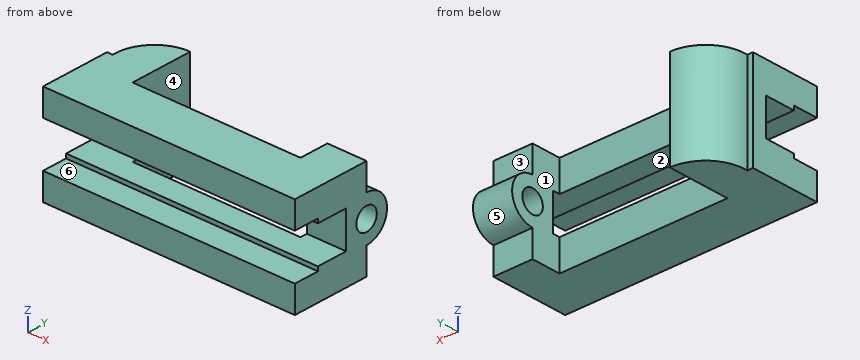
from build123d import *

# Parameters (mm, degrees)
BOSS_EXTRUDE1_DEPTH = 35
CUT_EXTRUDE1_DEPTH  = 201.062490237
SKETCH3_R           = 16
SKETCH3_R_2         = 8
BOSS_EXTRUDE2_DEPTH = 28
CUT_EXTRUDE2_REACH  = 202.062
SKETCH3_2_R         = 8


with BuildPart() as part:
    # Sketch1 → Boss-Extrude1 (new, symmetric)
    with BuildSketch(Plane.XY):
        with BuildLine():
            Line((0, 0), (180, 0))
            Line((180, 0), (180, 56))
            Line((180, 56), (152, 56))
            Line((152, 56), (152, 35))
            Line((152, 35), (32, 35))
            Line((32, 35), (32, 80))
            ThreePointArc((32, 80), (11.506098468, 71.078784028), (4.071519912, 50))
            Line((4.071519912, 50), (0, 50))
            Line((0, 50), (0, 0))
        make_face()
    extrude(amount=BOSS_EXTRUDE1_DEPTH, both=True)

    # Sketch2 → Cut-Extrude1 (cut, through all)
    with BuildSketch(Plane.ZY):
        Polygon((-16, 0), (-16, 18), (-13, 18), (-13, 40), (13, 40), (13, 18), (16, 18), (16, 0), align=None)
    extrude(amount=-CUT_EXTRUDE1_DEPTH, mode=Mode.SUBTRACT)

    # Sketch3 → Boss-Extrude2 (add)
    with BuildSketch(Plane(origin=(180, 0, 0), x_dir=(0, 0, -1), z_dir=(1, 0, 0))):
        with Locations((0, 56)):
            Circle(SKETCH3_R)
        with Locations((0, 56)):
            Circle(SKETCH3_R_2, mode=Mode.SUBTRACT)
    extrude(amount=-BOSS_EXTRUDE2_DEPTH)

    # Sketch3<2> → Cut-Extrude2 (cut, up to next)
    with BuildSketch(Plane(origin=(180, 0, 0), x_dir=(0, 0, -1), z_dir=(1, 0, 0)), mode=Mode.PRIVATE) as cut_extrude2_sk1:
        with Locations((0, 56)):
            Circle(SKETCH3_2_R)
    cut_extrude2_tool1 = extrude(cut_extrude2_sk1.sketch, amount=-CUT_EXTRUDE2_REACH, mode=Mode.PRIVATE) & part.part
    add(cut_extrude2_tool1.solids().sort_by_distance((180, 56, 0))[0], mode=Mode.SUBTRACT)


solid = part.part
Geometry check sheet. Reference: the model listing, model coordinates, mm. Face numbers are marked on the shaded views. A direction names the side the tool comes from. Coordinates: 2 decimals unless noted, no trailing zeros. Order: outer loops, then holes, each group sorted by start corner. A loop starts at its lowest first (then second) coordinate and runs counter-clockwise, first axis right, second up. Notation, with made-up numbers: (88.25, -3) - (99.25, -3) arc R25 cw to (99.25, 32) - close; hole circle Ø3 at (-22, 17). An arc over 180 degrees is marked (long way). One line per item, written item: value.
(1) Sectioned sample at D-D (z = 3.5). Enter the section's corners in (x, y), and give its area (3 significant figures).
Data:
outline: (0, 40) - (32, 40) - (32, 80) arc R28 ccw to (4.07, 50) - (0, 50) - close; (152, 40) - (180, 40) - (180, 48.81) - (152, 48.81) - close; (152, 63.19) - (180, 63.19) - (180, 71.61) - (152, 71.61) - close
area: 1,470 mm^2
(2) Depth check by flat-ended pin: pin 1 Ø2 at (x, z) = (83.5, -18.5) entering from -Y; pin 2 Ø8 at (x, z) = (47, 22.5) entering from +Y; pin 3 Ø0.9 at (x, z) = (77.5, -14) entering from -Y; pin 4 Ø15 at (x, z) = (165, -22) entering from +Y. Enter the tip coordinate at first touch or a pass-through.
Data:
pin 1: stops at y = 0
pin 2: stops at y = 35
pin 3: stops at y = 18
pin 4: stops at y = 62.76
(3) Sectioned sample at C-C (x = 77.5). Enter the section's corners in (y, z).
Data:
outline: (0, -35) - (35, -35) - (35, -13) - (18, -13) - (18, -16) - (0, -16) - close; (0, 16) - (18, 16) - (18, 13) - (35, 13) - (35, 35) - (0, 35) - close
(4) Release check for a two-part mould opening along Z. For the marked faces 4, 5 and 6 record: +Z half, -Z half, draft (parallel to the pull), parting line (faces both ways), or undercut.
Data:
face 4: draft
face 5: parting line
face 6: undercut
(5) Thickness scan on probe 1 along Y at (x, z) = (166.75, 0); probe 2 along Z at (x, y) = (131.5, 8); probe 3 along X at (y, z) = (36, 16.5). Record the ranges inside material, lowest first. Write a range as from..to.
Data:
probe 1: y = 40..48, 64..72
probe 2: z = -35..-16, 16..35
probe 3: x = 0..32, 152..180
(6) Sectioned sample at B-B (z = -20). Enter the section's corners in (x, y).
Data:
outline: (0, 0) - (180, 0) - (180, 56) - (152, 56) - (152, 35) - (32, 35) - (32, 80) arc R28 ccw to (4.07, 50) - (0, 50) - close
(7) Access from +Z, -Z, +X, -X, +Y, -Y to the whole of each face (thin tool, end or side, straight path). Record for the marked faces 1, 2 and 3.
Data:
face 1: +Z, -Z, +Y
face 2: +X, -X, -Y
face 3: +Z, +X, +Y
(8) Sectioned sample at A-A (y = 45). Enter the section's corners in (x, z).
Data:
outline: (0, -35) - (32, -35) - (32, 35) - (0, 35) - close; (152, -35) - (180, -35) - (180, 35) - (152, 35) - close
